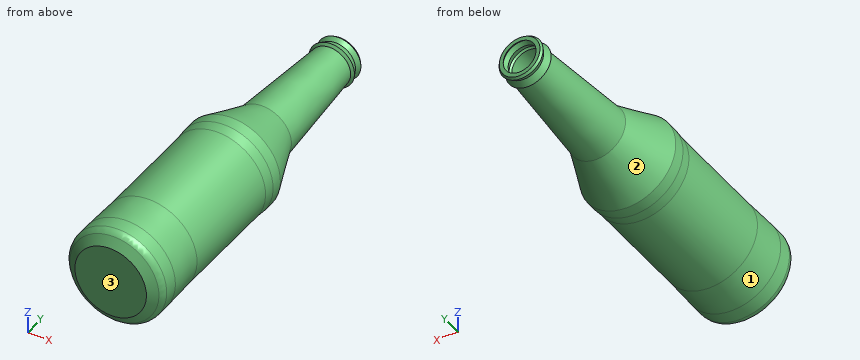
from build123d import *

# Parameters (mm, degrees)
FILLET2_R = 5


# Read off the part's stored shape, not the designer's step: Shell2
with BuildPart() as part:
    # Sketch1 → Revolve1 (revolve)
    with BuildSketch(Plane.XY, mode=Mode.PRIVATE) as revolve1_sk:
        Polygon((2.686675584, 14.691802026), (15.186675584, 14.691802026), (16.186675584, 13.242778256), (14.686675584, 10.327805917), (16.686675584, 6.141812908), (15.186675584, 4.836496853), (20.186675584, -61.163503147), (32.186675584, -91.163503147), (32.186675584, -98.267944917), (31.686675584, -104.864926562), (31.686675584, -171.996704513), (32.186675584, -193.979014243), (32.186675584, -205.127326289), (24.643709458, -210.308197974), (2.686675584, -210.308197974), align=None)
    revolve(revolve1_sk.sketch.rotate(Axis((2.686675584, -210.308197974, 0), (0, 1, 0)), 90), axis=Axis((2.686675584, -210.308197974, 0), (0, 1, 0)))

    # Fillet2
    fillet2_edges = [part.edges().sort_by_distance(p)[0] for p in [
        (2.686675584, -205.127326289, 29.5),
    ]]
    fillet(fillet2_edges, radius=FILLET2_R)

    # Shell2 outline → Shell2 (revolve, cut)
    with BuildSketch(Plane(origin=(2.686675584, 0, 0), x_dir=(1, 0, 0), z_dir=(0, 0, 1))):
        with BuildLine():
            Line((9.76769763, 10.360768085), (11.173521052, 13.092725677))
            Line((11.173521052, 13.092725677), (10.069966795, 14.691802026))
            Line((10.069966795, 14.691802026), (0, 14.691802026))
            Line((0, 14.691802026), (0, -208.308197974))
            Line((0, -208.308197974), (21.336339779, -208.308197974))
            Line((21.336339779, -208.308197974), (26.198491575, -204.968638423))
            ThreePointArc((26.198491575, -204.968638423), (27.154757496, -203.892994192), (27.5, -202.495760268))
            Line((27.5, -202.495760268), (27.5, -194.001756864))
            Line((27.5, -194.001756864), (27, -172.019447135))
            Line((27, -172.019447135), (27, -104.789242859))
            Line((27, -104.789242859), (27.5, -98.192261215))
            Line((27.5, -98.192261215), (27.5, -91.548667954))
            Line((27.5, -91.548667954), (15.528926693, -61.620984687))
            Line((15.528926693, -61.620984687), (10.429889715, 5.686303432))
            Line((10.429889715, 5.686303432), (11.539666623, 6.652043176))
            Line((11.539666623, 6.652043176), (9.76769763, 10.360768085))
        make_face()
    revolve(axis=Axis((2.686675584, 0, 0), (0, 1, 0)), mode=Mode.SUBTRACT)


solid = part.part
Geometry check sheet. Reference: the model listing, model coordinates, mm. Face numbers are marked on the shaded views. Give positions to 0.01 mm unless a question says otherwise; leave off trailing zeros. Loops run counter-clockwise (first coordinate to the right, second up) from the corner with the lowest first, then second, coordinate; pieces in that order, holes last. Notation, with made-up numbers: M 75,56.25 L 134,56.25 A20 ccw 134,79.25 Z; hole C 28.5,85 d2. An arc over 180 degrees is marked long. Answer as a JSON object with one key per item and string values. Group by question number.
Item 1: Material ranges on L1, parallel to X at y = -150, z = 0; L2, parallel to X at y = -200, z = 0; L3, parallel to Z at x = 4.5, y = -168, recorded low to high.
Item 2: Sectioned sample at A-A on y = -74. Record the boundary of the cut face in (x, z), plus the area to 3 significant figures.
Item 3: Mould release check, pull along Y, two halves, no side actions. Record for the marked faces 1, 2 and 3: pulls with the +Y half, pulls with the -Y half, needs draft (parallel to the pull), parting line crosses it, or undercut.
Item 4: Gauge pin test, flat ends, axial feed: pin 1 (1.5 mm diameter, centred on x = 7.5, y = -71.5, fed in from +Z); pin 2 (8 mm diameter, centred on x = 6, z = 0.5, fed in from +Y); pin 3 (6 mm diameter, centred on x = -10, y = -96.5, fed in from -Z). Record the tip position at first contact, or that the pin passes through.
Item 5: Sectioned sample at B-B on y = -7. Record the boundary of the cut face in (x, z).
Findings below:
{
 "1": {"L1": "-26.31 to -24.31, 29.69 to 31.69", "L2": "-26.81 to -24.81, 30.19 to 32.19", "L3": "-28.94 to -26.94, 26.94 to 28.94"},
 "2": {"outline": "C 2.69,0 d45.27; hole C 2.69,0 d40.96", "area": "292 mm2"},
 "3": {"face 1": "undercut", "face 2": "pulls with the +Y half", "face 3": "pulls with the -Y half"},
 "4": {"pin 1": "z = 21.44", "pin 2": "y = -208.31", "pin 3": "z = -27.86"},
 "5": {"outline": "C 2.69,0 d26.79; hole C 2.69,0 d22.78"}
}
